For this review, take the finished solid that the model builds, in its own axes (mm). A direction names the side the tool comes from. Give positions to 0.01 mm unless a question says otherwise; leave off trailing zeros. Loops run counter-clockwise (first coordinate to the right, second up) from the corner with the lowest first, then second, coordinate; pieces in that order, holes last. Notation, with made-up numbers: (50.25, 27) -> (101.25, 27) arc R19 ccw to (101.25, 64) -> close; hole circle Ø2 at (61.5, 11). An arc over 180 degrees is marked (long way). One line per question, with ' | ' between items. Start each with the question number.
(1) Wall thickness on probe 1 along X at (y, z) = (0, 7.25); probe 2 along Z at (x, y) = (5.5, 0.4): over which ranges is each line inside the solid? List them lowest first.
(2) Consider section B-B (x = 5.75). Write out the cut boundary in (y, z), and give its area (3 significant figures).
(3) Consider section A-A (y = 0.4). Write out the cut boundary in (x, z).
(4) Insertion check: P1, Ø0.9, axis at y = 0, z = 7, coming from the +X side; P2, Ø0.9, axis at y = 0.5, z = 7.5, coming from the -X side. Each pin has a flat end and moves straight along its axis. Give the tip position at first contact, or say it passes through.
(5) Tool access review of faces 1 (the flat face through (-4, 0, 8)), 2 (the flat face through (0, 0, -6)), 3 (the flat face through (6, 0, 6)): name each direction out of +Z, -Z, +X, -X, +Y, -Y from which nothing blocks a thin tool from reaching the whole face with its end or side.
from build123d import *

# Parameters (mm, degrees)
SKETCH6_W           = 15
SKETCH6_H           = 12
BOSS_EXTRUDE4_DEPTH = 1.5
SKETCH8_W           = 8
SKETCH8_H           = 3
BOSS_EXTRUDE5_DEPTH = 1.5


with BuildPart() as part:
    # Sketch6 → Boss-Extrude4 (new body, symmetric)
    with BuildSketch(Plane(origin=(0, 0, 0), x_dir=(1, 0, 0), z_dir=(0, 1, 0))):
        Rectangle(SKETCH6_W, SKETCH6_H)
    extrude(amount=BOSS_EXTRUDE4_DEPTH, both=True)

    # Sketch8 → Boss-Extrude5 (add, symmetric)
    with BuildSketch(Plane(origin=(0, 0, 0), x_dir=(1, 0, 0), z_dir=(0, 1, 0))):
        with Locations((0, -7.5)):
            Rectangle(SKETCH8_W, SKETCH8_H)
    extrude(amount=BOSS_EXTRUDE5_DEPTH, both=True)


solid = part.part
A:
1) probe 1: x = -4 to 4 | probe 2: z = -6 to 6
2) outline: (-1.5, -6) -> (1.5, -6) -> (1.5, 6) -> (-1.5, 6) -> close | area: 36.0 mm^2
3) outline: (-7.5, -6) -> (7.5, -6) -> (7.5, 6) -> (4, 6) -> (4, 9) -> (-4, 9) -> (-4, 6) -> (-7.5, 6) -> close
4) P1: stops at x = 4 | P2: stops at x = -4
5) face 1: +Z, -X, +Y, -Y | face 2: -Z, +X, -X, +Y, -Y | face 3: +Z, +X, +Y, -Y
